Here's how the part is built. I have some questions about the finished solid (model axes, mm). Face numbers are marked on the shaded views. A direction names the side the tool comes from. Give positions to 0.01 mm unless a question says otherwise; leave off trailing zeros. Loops run counter-clockwise (first coordinate to the right, second up) from the corner with the lowest first, then second, coordinate; pieces in that order, holes last.
Q1. For the marked faces 1, 2 and 3, which set-ups out of +Z, -Z, +X, -X, +Y, -Y let a thin tool reach every point of the face, with its end or its side?
Q2. If we section it at A-A (z = -6.05): Please give me the cut outline in (x, y), plus the area to 3 significant figures.
Q3. If we section it at C-C (y = 8.55): Please give me the cut outline in (x, z) (3 decimals), plus the area to 3 significant figures.
Q4. If we section it at B-B (x = 0.25): Please give me the cut outline in (y, z) (3 decimals), plus the area to 3 significant figures.
Q5. I need wall thicknesses on line 1 (Y direction, x = 2.5, z = -6); line 2 (X direction, y = 6, z = -3.5); line 3 (Y direction, x = -7.75, z = -3.5). Which ranges of each line are inside material? Lowest first, please.
Q6. Will these pins go through, and if not, where does the flat tip stop? P1, Ø4.5, axis at x = 4.5, y = 4, coming from the +Z side (3 decimals); P2, Ø2, axis at x = 4, y = 8.5, coming from the +Z side; P3, Ø6, axis at y = 2, z = -1, coming from the -X side; P4, Ø5, axis at x = -7.5, z = -8, coming from the -Y side.
Q7. We'd pull the mould along Y, two halves only. Please class the marked faces 4, 5 and 6: +Y half, -Y half, draft (parallel to the pull), parting line (faces both ways), or undercut.
Q8. If we section it at D-D (x = 2.25): Please give me the cut outline in (y, z) (3 decimals).
Autodesk Inventor part; units mm, degrees
ref_plane "YZ Plane" through (0, 0, 0) normal (1, 0, 0) x (0, 1, 0)
ref_plane "XZ Plane" through (0, 0, 0) normal (0, 1, 0) x (-1, 0, 0)
ref_plane "XY Plane" through (0, 0, 0) normal (0, 0, 1) x (1, 0, 0)
sketch "Sketch1" plane through (0, 0, 0) normal (1, 0, 0) x (0, 1, 0)
  line L0 (0, 0) -> (11.4, 0)
  line L1 (11.4, 0) -> (11.4, -12.1)
  line L2 (11.4, -12.1) -> (0, -12.1)
  line L3 (0, -12.1) -> (0, 0)
  arc A0 (11.4, -2.9512) -> (11.4, -9.1488) centre (12.8006, -6.05) ccw
  point P0 (3.5, -5)
  dimension "d0" = 11.4
  dimension "d1" = 12.1
  dimension "d2" = 6.1976
  dimension "d3" = 2.9512
  dimension "d29" = 2
extrude "Extrusion1" add sketch "Sketch1" along normal blind 6.35
extrude "Extrusion2" add sketch "Sketch1" against normal blind 11.43 contours L1 A0
sketch "Sketch3" plane through (0, 0, 0) normal (-1, 0, 0) x (0, 0, 1)
  line L0 (0, 11.4) -> (0, 0)
  line L1 (0, 0) -> (-12.1, 0)
  point P0 (-6.05, 5.7)
  dimension "d19" = 12.1
  dimension "d20" = 6.05
  dimension "d30" = 11.4
  dimension "d31" = 5.7
sketch "Sketch6" plane through (0, 0, 0) normal (0, 0, 1) x (1, 0, 0)
  line L0 (6.35, 5.7) -> (0, 5.7)
  line L1 (0, 0) -> (0, 11.4)
  line L2 (6.35, 11.4) -> (6.35, 0)
  line L3 (0, 0) -> (6.35, 0)
  line L4 (0, 11.4) -> (6.35, 11.4)
  dimension "d33" = 11.4
  dimension "d46" = 5.7
hole "Hole2" at (0, 5.7, -6.05) direction (1, 0, 0) diameter 4 end through all
extrude "Extrusion8" add sketch "Sketch6" along normal blind 3.175 contours L0 L1 L4 L2
sketch "Sketch7" plane through (0, 0, 3.175) normal (0, 0, 1) x (1, 0, 0)
  line L0 (6.35, 11.4) -> (0, 11.4)
  line L1 (6.35, 5.7) -> (6.35, 11.4)
  point P0 (0, 0)
  point P1 (3.175, 8.55)
  dimension "d50" = 6.35
  dimension "d51" = 5.7
  dimension "d52" = 2.85
  dimension "d53" = 3.175
sketch "Sketch8" plane through (0, 0, 3.175) normal (0, 0, 1) x (1, 0, 0)
  circle A0 centre (3.175, 8.55) radius 2
  line L0 (6.35, 11.4) -> (0, 11.4)
  line L1 (6.35, 5.7) -> (6.35, 11.4)
  point P0 (0, 0)
  dimension "d63" = 2.85
  dimension "d64" = 3.175
  dimension "d65" = 4
extrude "Extrusion9" cut sketch "Sketch8" against normal up to surface (3.175 mm away)
thread "Thread2"
equation "\"d3\" = -0.5 * d2 + 0.5 * d1"
equation "\"d46\" = 0.5 * d33"
equation "\"d63\" = d52"
equation "\"d64\" = d53"
properties part number "end peice for slides"
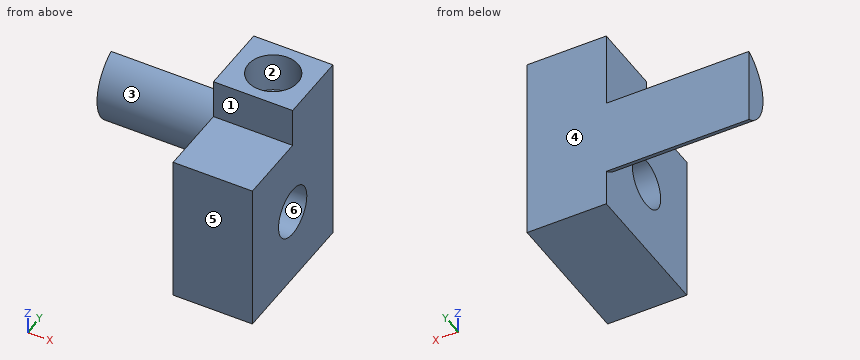
Check sheet entries:
1. face 1: +Z, +X, -X, -Y
1. face 2: +Z
1. face 3: -X, -Y
2. outline: (-11.43, 9.4) - (0, 9.4) - (0, 7.7) - (6.35, 7.7) - (6.35, 11.4) - (-11.43, 11.4) - close; (0, 0) - (6.35, 0) - (6.35, 3.7) - (0, 3.7) - close
2. area: 69.9 mm2
3. outline: (0, -12.1) - (6.35, -12.1) - (6.35, 3.175) - (5.175, 3.175) - (5.175, 0) - (1.175, 0) - (1.175, 3.175) - (0, 3.175) - close
3. area: 84.3 mm2
4. outline: (0, -12.1) - (11.4, -12.1) - (11.4, 3.175) - (5.7, 3.175) - (5.7, 0) - (0, 0) - close; hole circle Ø4 at (5.7, -6.05)
4. area: 143 mm2
5. line 1: y = 0 to 3.7, 7.7 to 11.4
5. line 2: x = 0 to 6.35
5. line 3: y = 10.55 to 11.4
6. P1: stops at z = 3.175
6. P2: stops at z = 0
6. P3: stops at x = 0
6. P4: stops at y = 9.4
7. face 4: +Y half
7. face 5: -Y half
7. face 6: undercut
8. outline: (0, -12.1) - (11.4, -12.1) - (11.4, 3.175) - (10.323, 3.175) - (10.323, 0) - (6.777, 0) - (6.777, 3.175) - (5.7, 3.175) - (5.7, 0) - (0, 0) - close; hole circle Ø4 at (5.7, -6.05)
